Can you work these out from the drawing? Everything is in mm from the part's minimum corner. A direction names the side the tool comes from. Coordinates: 2 decimals unless noted, no trailing zeros. Write each loop counter-clockwise with the first axis right and the second up, starting at its lowest first coordinate (ties: lowest second). Pieces come first, ordered by that corner, then holes.
(1) Imagine slicing it at A-A, the plane y = 22.5. State how many separate pieces and enclosed holes the cut face has, plus the area to 3 significant figures.
(2) Please list where these lines run through material, in increasing order: probe 1 along Y at (x, z) = (7.25, 23); probe 2 along X at (y, z) = (22.5, 39); probe 3 along X at (y, z) = (22.5, 11.65).
(3) Thinking about a two-plate mould opening in X: for the marked faces 1, 2 and 3, which applies, released by +X, released by -X, zero draft, split by the parting line, or undercut?
(4) Imagine slicing it at B-B, the plane z = 40.5. List the corners of the cut face in (x, y) for me, plus the area to 3 significant figures.
(5) Imagine slicing it at D-D, the plane x = 16.75. List the corners of the cut face in (y, z) for me.
(6) Imagine slicing it at C-C, the plane x = 20. List the corners of the cut face in (y, z) for me.
(7) Which directions (+Z, -Z, +X, -X, +Y, -Y) give clear straight access to the entire face, cutting with the end or side of a thin tool? Please do the marked faces 4, 5, 6 and 7.
(8) For pin 1 Ø3 at (x, y) = (14.5, 22) entering from -Z; pin 2 Ø6 at (x, z) = (6, 13.5) entering from -Y; pin 3 Ø5 at (x, y) = (20, 22.5) entering from +Z; pin 4 Ø2.5 at (x, y) = (20, 22.5) entering from +Z, each with a flat end and sliding along its axis, tell me the tip position at first contact or that it passes through.
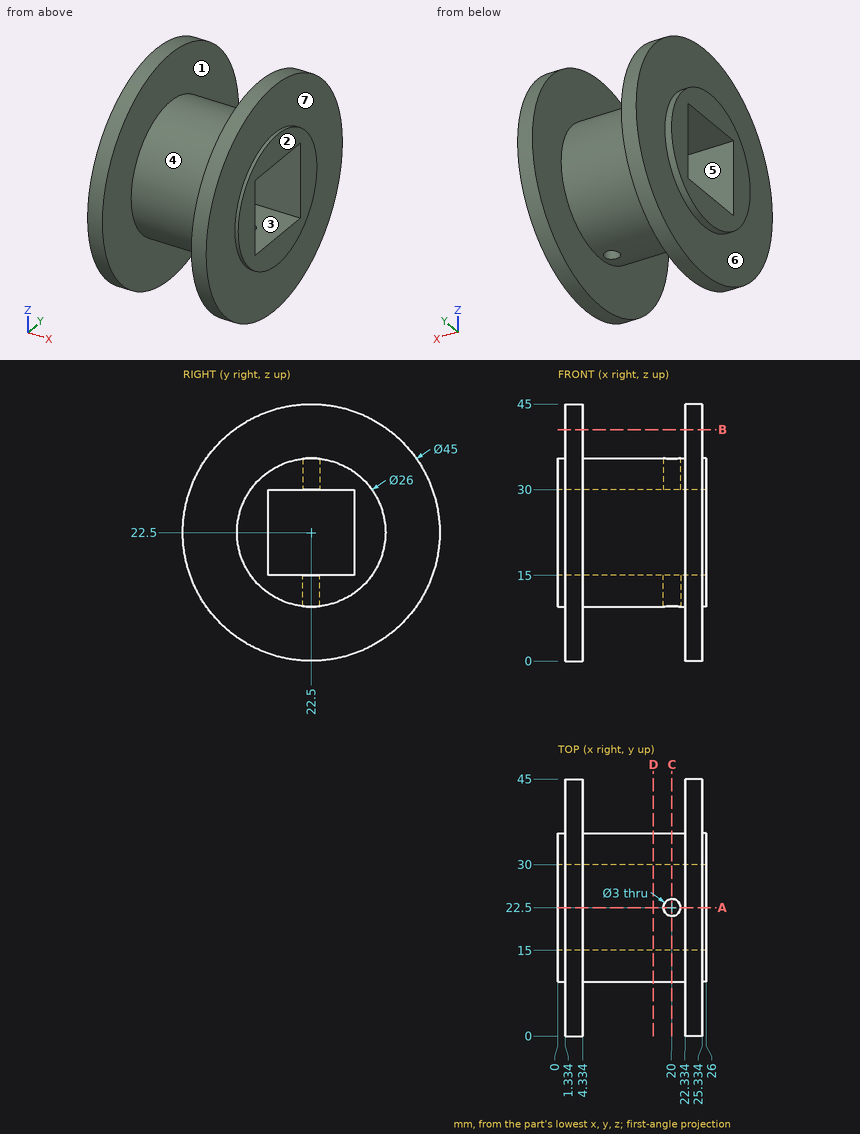
Recorded:
1. separate pieces: 4
1. enclosed holes: 0
1. area: 367 mm2
2. probe 1: y = 9.51 to 15, 30 to 35.49
2. probe 2: x = 1.33 to 4.33, 22.33 to 25.33
2. probe 3: x = 0 to 18.5, 21.5 to 26
3. face 1: undercut
3. face 2: released by +X
3. face 3: zero draft
4. outline: (1.33, 9) - (4.33, 9) - (4.33, 36) - (1.33, 36) - close; (22.33, 9) - (25.33, 9) - (25.33, 36) - (22.33, 36) - close
4. area: 162 mm2
5. outline: circle Ø26 at (22.5, 22.5); hole (15, 15) - (30, 15) - (30, 30) - (15, 30) - close
6. outline: (15, 15) - (15, 30) - (21, 30) - (21, 35.41) arc R13 ccw to (21, 9.59) - (21, 15) - close; (24, 9.59) arc R13 ccw to (24, 35.41) - (24, 30) - (30, 30) - (30, 15) - (24, 15) - close
7. face 4: none
7. face 5: +X, -X
7. face 6: -X
7. face 7: +X
8. pin 1: stops at z = 9.5
8. pin 2: stops at y = 0.96
8. pin 3: stops at z = 45
8. pin 4: passes through
